Answer from the drawing. Dimensions are ordinates in mm from the lowest x, y and z of the part. Give positions to 0.01 mm unless a question says otherwise; leave off trailing zeros. Loops run counter-clockwise (first coordinate to the right, second up) from the corner with the lowest first, then second, coordinate; pieces in that order, holes last. Notation, with made-up numbers: (17, 45.25) - (21, 45.25) arc R22 ccw to (21, 56.25) - close; hole circle Ø8 at (-32, 9.25). An arc over 180 degrees is marked (long way). One line per question, with ' | ' between items. Start each with the question number.
1. Section A-A (z = 35) is taken. Determine the outline of the cut face in (x, y) (3 decimals), plus the area to 3 significant figures.
2. For a pull along Z with two mould halves and no side action, classify the marked faces 1, 2, 3 and 4 as released by +Z, released by -Z, zero draft, split by the parting line, or undercut.
3. This flat-tipped pin is pushed along its axis until it touches: pin 1 (4 mm diameter, centred on x = 3, z = 33, fed in from -Y). Where does it stop, or does it pass through?
4. Section C-C (y = 20) is taken. Determine the outline of the cut face in (x, z) (3 decimals).
5. Section B-B (x = 11.25) is taken. Determine the outline of the cut face in (y, z) (3 decimals).
6. Find the intervals of material crossed by line 1 (X direction, y = 47.5, z = 9) (3 decimals); line 2 (Z direction, x = 21, y = 94) (3 decimals), in increasing order.
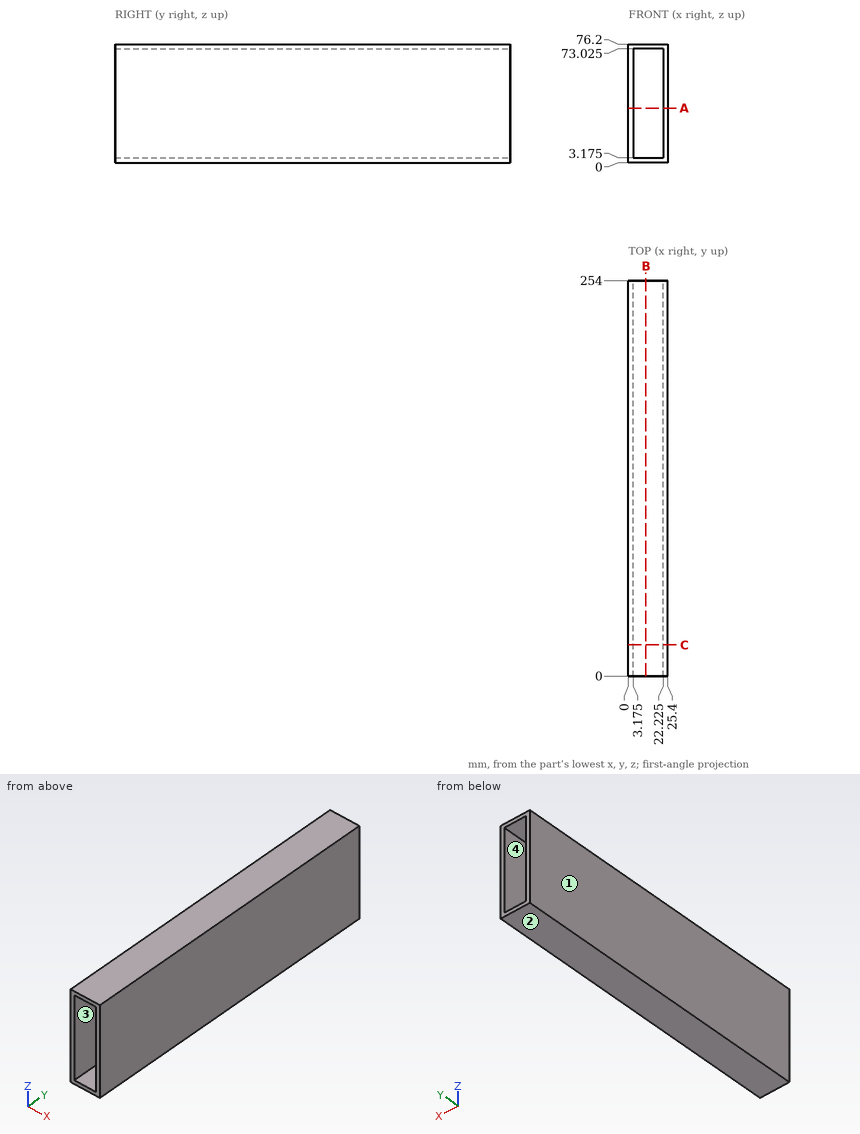
Conclusion:
1) outline: (0, 0) - (3.175, 0) - (3.175, 254) - (0, 254) - close; (22.225, 0) - (25.4, 0) - (25.4, 254) - (22.225, 254) - close | area: 1,610 mm²
2) face 1: zero draft | face 2: released by -Z | face 3: undercut | face 4: undercut
3) pin 1: y = 0
4) outline: (0, 0) - (25.4, 0) - (25.4, 76.2) - (0, 76.2) - close; hole (3.175, 3.175) - (22.225, 3.175) - (22.225, 73.025) - (3.175, 73.025) - close
5) outline: (0, 0) - (254, 0) - (254, 3.175) - (0, 3.175) - close; (0, 73.025) - (254, 73.025) - (254, 76.2) - (0, 76.2) - close
6) line 1: 0 to 3.175, 22.225 to 25.4 | line 2: 0 to 3.175, 73.025 to 76.2
